Source: three-view drawing plus pictorial views. Frame: mm from the lowest corner of the part. Coordinates: 2 decimals unless noted, no trailing zeros. Write each loop counter-clockwise with the first axis right and the second up, starting at its lowest first coordinate (ties: lowest second). Pieces come first, ordered by that corner, then holes. Notation, with made-up numbers: (-30.5, 54.25) - (-21.5, 54.25) arc R18 cw to (-21.5, 61.25) - close; hole circle Ø4 at (-19.5, 13). An arc over 180 degrees is marked (long way). Put each result on its own line as item: value.
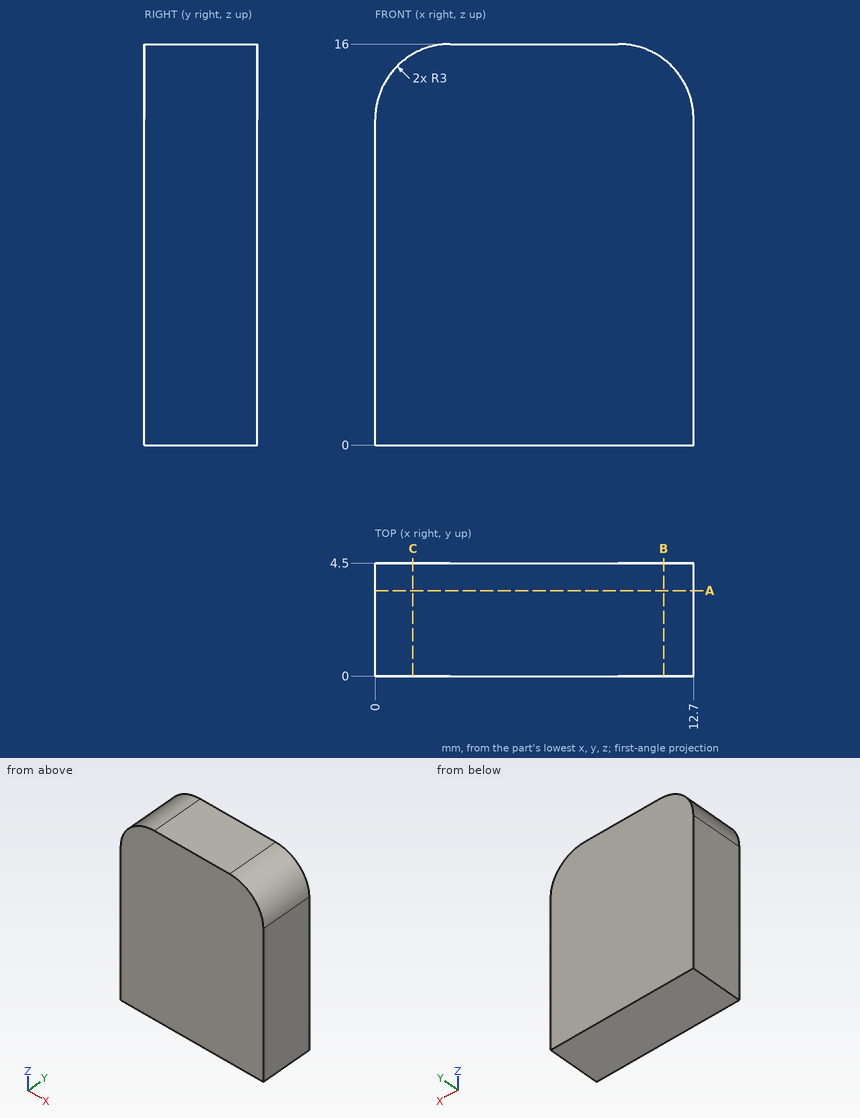
1. Section query A-A (y = 3.4). Return loops of the section in (x, z), then the cut area to 3 significant figures.
Answer below:
outline: (0, 0) - (12.7, 0) - (12.7, 13) arc R3 ccw to (9.7, 16) - (3, 16) arc R3 ccw to (0, 13) - close
area: 199 mm²
2. Section query C-C (x = 1.5). Return loops of the section in (y, z), then the cut area to 3 significant figures.
Answer below:
outline: (0, 0) - (4.5, 0) - (4.5, 15.6) - (0, 15.6) - close
area: 70.2 mm²
3. Ray query, probe 1 along Z at (x, y) = (12, 2); probe 2 along X at (y, z) = (0.5, 15); probe 3 along Z at (x, y) = (1.75, 2.1). Return the intervals inside material, ascending. Write a range as from..to.
Answer below:
probe 1: z = 0..14.93
probe 2: x = 0.76..11.94
probe 3: z = 0..15.73
4. Section query B-B (x = 11.5). Return loops of the section in (y, z).
Answer below:
outline: (0, 0) - (4.5, 0) - (4.5, 15.4) - (0, 15.4) - close
